```python
from build123d import *

# Parameters (mm, degrees)
BOSS_EXTRUDE1_DEPTH = 19.05
SKETCH2_R           = 2.5796875
CUT_EXTRUDE1_DEPTH  = 20.05
SKETCH3_R           = 6.604
CUT_EXTRUDE2_DEPTH  = 6.604
CHAMFER1_SIZE       = 0.5
FILLET1_R           = 3.175
FILLET2_R           = 1


with BuildPart() as part:
    # Sketch1 → Boss-Extrude1 (new body)
    with BuildSketch(Plane(origin=(0, 0, 0), x_dir=(1, 0, 0), z_dir=(0, 1, 0))):
        with BuildLine():
            Line((6.35, 0), (44.45, 0))
            ThreePointArc((44.45, 0), (48.940128061, 1.859871939), (50.8, 6.35))
            Line((50.8, 6.35), (50.8, 25.4))
            Line((50.8, 25.4), (0, 25.4))
            Line((0, 25.4), (0, 6.35))
            ThreePointArc((0, 6.35), (1.859871939, 1.859871939), (6.35, 0))
        make_face()
    extrude(amount=BOSS_EXTRUDE1_DEPTH)

    # Sketch2 → Cut-Extrude1 (cut, through all)
    with BuildSketch(Plane(origin=(0, 19.05, 0), x_dir=(1, 0, 0), z_dir=(0, 1, 0))):
        with Locations(Location((9.525, 12.7, 0), (0, 0, 270))):  # turned: the seam where the file's is
            Circle(SKETCH2_R)
        with Locations(Location((41.275, 12.7, 0), (0, 0, 90))):  # turned: the seam where the file's is
            Circle(SKETCH2_R)
    extrude(amount=-CUT_EXTRUDE1_DEPTH, mode=Mode.SUBTRACT)

    # Sketch3 → Cut-Extrude2 (cut)
    with BuildSketch(Plane(origin=(0, 0, -25.4), x_dir=(-1, 0, 0), z_dir=(0, 0, -1))):
        with Locations((-41.275, 9.525)):
            Circle(SKETCH3_R)
        with Locations(Location((-9.525, 9.525, 0), (0, 0, 180))):  # turned: the seam where the file's is
            Circle(SKETCH3_R)
    extrude(amount=-CUT_EXTRUDE2_DEPTH, mode=Mode.SUBTRACT)

    # Chamfer1
    chamfer1_edges = [part.edges().sort_by_distance(p)[0] for p in [
        (9.525, 0, -15.2796875),
        (9.525, 19.05, -15.2796875),
        (41.275, 0, -10.1203125),
        (41.275, 19.05, -10.1203125),
        (47.879, 9.525, -25.4),
        (2.921, 9.525, -25.4),
    ]]
    chamfer(chamfer1_edges, length=CHAMFER1_SIZE)

    # Fillet1
    fillet1_edges = [part.edges().sort_by_distance(p)[0] for p in [
        (48.940128061, 0, -1.859871939),
        (25.4, 0, 0),
        (1.859871939, 0, -1.859871939),
        (0, 0, -15.875),
        (50.8, 0, -15.875),
    ]]
    fillet(fillet1_edges, radius=FILLET1_R)

    # Fillet2
    fillet2_edges = [part.edges().sort_by_distance(p)[0] for p in [
        (0, 19.05, -15.875),
        (0, 11.1125, -25.4),
        (50.8, 11.1125, -25.4),
        (1.859871939, 19.05, -1.859871939),
        (25.4, 19.05, 0),
        (48.940128061, 19.05, -1.859871939),
        (50.8, 19.05, -15.875),
        (25.4, 0, -25.4),
        (49.87006403, 0.92993597, -25.4),
        (0.92993597, 0.92993597, -25.4),
        (25.4, 19.05, -25.4),
    ]]
    fillet(fillet2_edges, radius=FILLET2_R)


solid = part.part
```
Design review of the part built by this model. Coordinates are the model's own, in mm. A direction names the side the tool comes from. Round coordinates to 2 decimals unless told otherwise and drop trailing zeros. Write each loop counter-clockwise with the first axis right and the second up, starting at its lowest first coordinate (ties: lowest second). Pieces come first, ordered by that corner, then holes.
Item 1: For probe 1 along X at (y, z) = (6.5, -12.7); probe 2 along X at (y, z) = (10, -19.75); probe 3 along Z at (x, y) = (9.5, 18), list the stretches that pass through material, from the lowest coordinate up.
Item 2: We need section C-C on y = 13.25. State how many separate pieces and enclosed holes the cut face has, and give its area (3 significant figures).
Item 3: Clearance check with flat-ended pins moving along their axes: pin 1 Ø8.5 at (x, z) = (9.525, -12.7) entering from -Y; pin 2 Ø6.5 at (x, y) = (44.5, 9.5) entering from -Z. State where each tip first meets the part, or that it passes through.
Item 4: We need section B-B on z = -22.25. Write out the cut boundary in (x, y) (3 decimals), and give its area (3 significant figures).
Item 5: For faces 1 (the cylindrical face through (49.85, 0.91, -15.5)), 2 (the cylindrical face through (35.175, 6.996, -21.891)), list the 3-axis set-ups (+Z, -Z, +X, -X, +Y, -Y) from which the entire face can be reached by the end or side of a thin tool; tool diameter is ignored.
Item 6: The part is to be moulded in two halves that separate along Z. For faces 3 (the flat face through (25, 0, -14)), 4 (the flat face through (25, 11, 0)), 5 (the cylindrical face through (39.1, 9.65, -14.09)), say which applies: +Z half, -Z half, draft (parallel to the pull), parting line (faces both ways), or undercut.
Item 7: We need section A-A on z = -12.7. Write out the cut boundary in (x, y) (3 decimals).
Returned:
1. probe 1: x = 0 to 6.95, 12.1 to 38.7, 43.85 to 50.8
1. probe 2: x = 0 to 2.94, 16.11 to 34.69, 47.86 to 50.8
1. probe 3: z = -25.4 to -15.28, -10.12 to 0
2. separate pieces: 1
2. enclosed holes: 2
2. area: 1,090 mm2
3. pin 1: stops at y = 0
3. pin 2: stops at z = -18.8
4. outline: (0, 3.175) arc R3.175 ccw to (3.175, 0) - (47.625, 0) arc R3.175 ccw to (50.8, 3.175) - (50.8, 18.05) arc R1 ccw to (49.8, 19.05) - (1, 19.05) arc R1 ccw to (0, 18.05) - close; hole circle Ø13.208 at (9.525, 9.525); hole circle Ø13.208 at (41.275, 9.525)
4. area: 689 mm2
5. face 1: +Z, -Z, +X, -Y
5. face 2: -Z
6. face 3: draft
6. face 4: +Z half
6. face 5: undercut
7. outline: (0, 3.175) arc R3.175 ccw to (3.175, 0) - (6.445, 0) - (6.945, 0.5) - (6.945, 18.55) - (6.445, 19.05) - (1, 19.05) arc R1 ccw to (0, 18.05) - close; (12.105, 0.5) - (12.605, 0) - (38.195, 0) - (38.695, 0.5) - (38.695, 18.55) - (38.195, 19.05) - (12.605, 19.05) - (12.105, 18.55) - close; (43.855, 0.5) - (44.355, 0) - (47.625, 0) arc R3.175 ccw to (50.8, 3.175) - (50.8, 18.05) arc R1 ccw to (49.8, 19.05) - (44.355, 19.05) - (43.855, 18.55) - close
